Can you work these out from the model? Positions are in its coordinate system, mm. A direction names the side the tool comes from. Give positions to 0.01 mm unless a question says otherwise; leave off trailing zeros. Write each loop counter-clockwise with the first axis right and the second up, starting at its lowest first coordinate (ties: lowest second). Pieces come first, ordered by that corner, then holes. Notation, with made-up numbers: (-20.75, 86.25) -> (23.25, 86.25) arc R23 cw to (23.25, 94.25) -> close; hole circle Ø11 at (3, 33.25). An arc over 180 degrees is marked (long way). One line per item, written item: value.
Autodesk Inventor part; units mm, degrees
ref_plane "YZ Plane" through (0, 0, 0) normal (1, 0, 0) x (0, 1, 0)
ref_plane "XZ Plane" through (0, 0, 0) normal (0, 1, 0) x (-1, 0, 0)
ref_plane "XY Plane" through (0, 0, 0) normal (0, 0, 1) x (1, 0, 0)
sketch "Sketch1" plane through (0, 0, 0) normal (0, 0, 1) x (1, 0, 0)
  arc A0 (0, 31.75) -> (0, -31.75) centre (0, 0) ccw
  arc A1 (508, -31.75) -> (508, 31.75) centre (508, 0) ccw
  line L0 (508, -31.75) -> (25.9095, -31.75)
  line L1 (0, 31.75) -> (12.9547, 31.75)
  arc A2 (0, 36.75) -> (0, -36.75) centre (0, 0) ccw
  line L2 (0, 36.75) -> (508, 36.75)
  line L3 (508, -36.75) -> (0, -36.75)
  arc A3 (508, -36.75) -> (508, 36.75) centre (508, 0) ccw
  line L4 (495.0453, 31.75) -> (508, 31.75)
  line L5 (12.9547, 31.75) -> (495.0453, 31.75)
  line L6 (25.9095, -31.75) -> (0, -31.75)
  dimension "d0" = 63.5
  dimension "d1" = 508
  dimension "d2" = 73.5
extrude "Extrusion1" add sketch "Sketch1" along normal blind 150
properties part number "banda1"
1) We'd pull the mould along X, two halves only. Please class faces 1 (the face through (-36.74, -0.81, 73.95)), 2 (the face through (258, -36.75, 74)), 3 (the face through (-31.742, -0.698, 73.95)), 4 (the face through (539.742, 0.698, 73.95)): released by +X, released by -X, zero draft, split by the parting line, or undercut.
Answer list:
face 1: released by -X
face 2: zero draft
face 3: undercut
face 4: undercut
2) If we section it at C-C (z = 58.5): Write out the boundary of the cut face in (x, y).
Answer list:
outline: (0, -36.75) -> (508, -36.75) arc R36.75 ccw to (508, 36.75) -> (0, 36.75) arc R36.75 ccw to start; hole (0, -31.75) -> (508, -31.75) arc R31.75 ccw to (508, 31.75) -> (0, 31.75) arc R31.75 ccw to start
3) If we section it at B-B (x = 397.5): Write out the boundary of the cut face in (y, z), and give its area (3 significant figures).
Answer list:
outline: (-36.75, 0) -> (-31.75, 0) -> (-31.75, 150) -> (-36.75, 150) -> close; (31.75, 0) -> (36.75, 0) -> (36.75, 150) -> (31.75, 150) -> close
area: 1,500 mm^2
4) For faces 5 (the face through (250, 31.75, 74)), 6 (the face through (544.74, 0.81, 73.95)), which set-ups out of +Z, -Z, +X, -X, +Y, -Y let a thin tool reach every point of the face, with its end or its side?
Answer list:
face 5: +Z, -Z
face 6: +Z, -Z, +X
5) I need wall thicknesses on L1, parallel to Y at x = 239, z = 65; L2, parallel to X at y = 14, z = 11.5; L3, parallel to X at y = -26, z = 7. Which ranges of each line are inside material? Lowest first, please.
Answer list:
L1: y = -36.75 to -31.75, 31.75 to 36.75
L2: x = -33.98 to -28.5, 536.5 to 541.98
L3: x = -25.97 to -18.22, 526.22 to 533.97
6) If we section it at A-A (y = 0): Write out the boundary of the cut face in (x, z).
Answer list:
outline: (-36.75, 0) -> (-31.75, 0) -> (-31.75, 150) -> (-36.75, 150) -> close; (539.75, 0) -> (544.75, 0) -> (544.75, 150) -> (539.75, 150) -> close
7) Will these pins go through, and if not, where does the flat tip stop? pin 1 (10 mm diameter, centred on y = -21.5, z = 23, fed in from -X); pin 2 (2 mm diameter, centred on y = 25.5, z = 119.5, fed in from -X); pin 3 (2 mm diameter, centred on y = -15.5, z = 133, fed in from -X).
Answer list:
pin 1: stops at x = -32.84
pin 2: stops at x = -27.39
pin 3: stops at x = -33.77
